```python
from build123d import *

# Parameters (mm, degrees)
SKETCH2_R              = 1.25
CUT_EXTRUDE_M2_5_DEPTH = 5
CIRPATTERN1_COUNT      = 4


with BuildPart() as part:
    # Sketch1 → Revolve1 (revolve)
    with BuildSketch(Plane.XY, mode=Mode.PRIVATE) as revolve1_sk:
        Polygon((-8.5, 4.25), (-5, 4.25), (-5, 7), (-12.5, 7), (-12.5, 6), (-10.5, 6), (-10.5, 5), (-8.5, 5), align=None)
        Polygon((-2.5, 4.25), (-2.5, 16.5), (-5, 16.5), (-5, 7), (-5, 4.25), align=None)
        Polygon((2.5, 20.95), (-2.5, 20.95), (-2.5, 16.5), (-2.5, 4.25), (2.5, 4.25), (2.5, 7), align=None)
        Polygon((15.5, 7), (2.5, 7), (2.5, 4.25), (11.5, 4.25), (11.5, 5), (13.5, 5), (13.5, 6), (15.5, 6), align=None)
    revolve(revolve1_sk.sketch.rotate(Axis((0, 0, 0), (1, 0, 0)), 90), axis=Axis((0, 0, 0), (1, 0, 0)))

    # Sketch2 → Cut-Extrude M2.5 (cut)
    with BuildSketch(Plane.ZY.offset(5)):
        with Locations((9.192388155, 9.192388155)):
            Circle(SKETCH2_R)
    cut_extrude_m2_5 = extrude(amount=-CUT_EXTRUDE_M2_5_DEPTH, mode=Mode.SUBTRACT)

    # CirPattern1: Cut-Extrude M2.5 ×4 about axis
    cirpattern1_axis = Axis((0, 0, 0), (1, 0, 0))
    for i in range(1, CIRPATTERN1_COUNT):
        add(cut_extrude_m2_5.rotate(cirpattern1_axis, i * 360 / CIRPATTERN1_COUNT), mode=Mode.SUBTRACT)


solid = part.part
```
The listing builds one solid part. Answer for the finished solid, in the listing's coordinates (mm). A direction names the side the tool comes from. Give positions to 0.01 mm unless a question says otherwise; leave off trailing zeros. Loops run counter-clockwise (first coordinate to the right, second up) from the corner with the lowest first, then second, coordinate; pieces in that order, holes last. Notation, with made-up numbers: (-20.5, -9) - (30.5, -9) arc R28 ccw to (30.5, 28) - close; hole circle Ø6 at (47.5, 75). An arc over 180 degrees is marked (long way). Return JSON: item names as keys, results as strings. Group by question number.
1. Straight lines are drawn through the part: line 1 (Y direction, x = -0.5, z = 0); line 2 (Y direction, x = -1.5, z = -10); line 3 (Y direction, x = -1, z = -9). For each, find the intervals that lie inside material, in ascending order. Write a range as [from, to].
2. Given pin 1 Ø8 at (y, z) = (-1, -11.5) entering from +X; pin 2 Ø11.5 at (y, z) = (0, 0) entering from -X; pin 3 Ø3 at (y, z) = (-9, 9) entering from -X, each flat-ended and moving along its own axis, determine where each tip first touches the part or whether it passes through.
3. Find section B-B (z = 8.5). Write down the section's boundary in (x, y).
4. Find section A-A (x = 1.75). Write down the section's boundary in (y, z), then the cut area to 3 significant figures.
5. Which of the six approach directions +Z, -Z, +X, -X, +Y, -Y give full straight-line access (tool end or side, diameter ignored) to faces 5 (the flat face through (2.5, 0, -9)), 6 (the cylindrical face through (1.64, -4.214, -0.553)), 7 (the flat face through (0, -9, -9))?
6. Find section C-C (y = 12). Write down the section's boundary in (x, z).
7. Determine the mould class of faces 1 (the flat face through (15.5, -2, -6)), 2 (the cylindrical face through (-0.035, 20.452, -4.542)), 3 (the cylindrical face through (-9, 0, -5)), 4 (the flat face through (13.5, -4, 4)) for opening direction Z: pulls with the +Z half, pulls with the -Z half, needs draft (parallel to the pull), parting line crosses it, or undercut.
8. Find section D-D (x = -7.25). Write down the section's boundary in (y, z).
Verdict:
{
 "1": {"line 1": "y = [-20.95, -4.25], [4.25, 20.95]", "line 2": "y = [-18.41, -10.15], [-8.24, 8.24], [10.15, 18.41]", "line 3": "y = [-18.92, -10.43], [-7.96, 7.96], [10.43, 18.92]"},
 "2": {"pin 1": "stops at x = 2.5", "pin 2": "stops at x = -10.5", "pin 3": "stops at x = -5"},
 "3": {"outline": "(-5, -14.14) - (-2.5, -14.14) - (-2.5, -19.15) - (2.5, -19.15) - (2.5, 19.15) - (-2.5, 19.15) - (-2.5, 14.14) - (-5, 14.14) - (-5, 10.23) - (0, 10.23) - (0, 8.15) - (-5, 8.15) - (-5, -8.15) - (0, -8.15) - (0, -10.23) - (-5, -10.23) - close"},
 "4": {"outline": "circle Ø41.9 at (0, 0); hole circle Ø8.5 at (0, 0)", "area": "1,320 mm^2"},
 "5": {"face 5": "+X", "face 6": "+X, -X", "face 7": "-X"},
 "6": {"outline": "(-5, -11.32) - (-2.5, -11.32) - (-2.5, -17.17) - (2.5, -17.17) - (2.5, 17.17) - (-2.5, 17.17) - (-2.5, 11.32) - (-5, 11.32) - close"},
 "7": {"face 1": "needs draft", "face 2": "parting line crosses it", "face 3": "undercut", "face 4": "undercut"},
 "8": {"outline": "circle Ø14 at (0, 0); hole circle Ø8.5 at (0, 0)"}
}
